Verification items for the finished model (mm, model axes). Face numbers are marked on the shaded views. A direction names the side the tool comes from. Give positions to 0.01 mm unless a question says otherwise; leave off trailing zeros. Order: outer loops, then holes, each group sorted by start corner. A loop starts at its lowest first (then second) coordinate and runs counter-clockwise, first axis right, second up. Notation, with made-up numbers: M -25,18 L 19,18 A24 ccw 19,45 Z; hole C 52.5,83 d1. An arc over 180 degrees is marked long. Answer as a JSON object with one key per item and string values.
```python
from build123d import *

# Parameters (mm, degrees)
SKETCH_R                       = 2.25
SKETCH_R_2                     = 1.75
PAD_DEPTH                      = 12
POCKET_DEPTH                   = 2
SKETCH002_R                    = 2.25
POCKET002_DEPTH                = 20.001
PART_MIRRORING_PLACEMENT_ANGLE = 180
SKETCH003_R                    = 3
POCKET003_DEPTH                = 8
SKETCH004_R                    = 3.75
POCKET004_DEPTH                = 10


with BuildPart() as pocket002:
    # Sketch → Pad (new body)
    with BuildSketch(Plane.XY):
        Polygon((0, -20), (40, -20), (40, 20), (-20, 20), (-20, 0), (0, 0), align=None)
        with Locations((18, 8)):
            Circle(SKETCH_R, mode=Mode.SUBTRACT)
        with Locations((13, -10)):
            Circle(SKETCH_R, mode=Mode.SUBTRACT)
        with Locations((35, 15)):
            Circle(SKETCH_R_2, mode=Mode.SUBTRACT)
        with Locations((28, -10)):
            Circle(SKETCH_R, mode=Mode.SUBTRACT)
    extrude(amount=PAD_DEPTH)

    # Sketch001 → Pocket (cut)
    with BuildSketch(Plane.XY.offset(12)):
        with BuildLine():
            Line((46, 10), (29, 10))
            ThreePointArc((29, 10), (25.778175, 17.778175), (18, 21))
            Line((18, 21), (0, 21))
            Line((0, 21), (0, -23))
            Line((0, -23), (46, -23))
            Line((46, -23), (46, -12))
            Line((28.629901, -14.455696), (46, -12))
            ThreePointArc((28.629901, -5.544304), (23.5, -10), (28.629901, -14.455696))
            Line((28.629901, -5.544304), (46, -8))
            Line((46, -8), (46, 10))
        make_face()
    extrude(amount=-POCKET_DEPTH, mode=Mode.SUBTRACT)

    # Sketch002 → Pocket002 (cut, through all)
    with BuildSketch(Plane.XZ):
        with Locations((-10, 6)):
            Circle(SKETCH002_R)
    extrude(amount=-POCKET002_DEPTH, mode=Mode.SUBTRACT)


with BuildPart() as pocket004:
    # Part__Mirroring: instance of Pocket002
    add(pocket002.part.mirror(Plane(origin=(10, -0.411961, 0), x_dir=(0, 1, 0), z_dir=(0, 0, 1))))


with BuildPart() as pocket004_1:
    # Part__Mirroring placement: moved
    add(pocket004.part.rotate(Axis((0, 0, 0), (1, 0, 0)), PART_MIRRORING_PLACEMENT_ANGLE))

    # Sketch003 → Pocket003 (cut)
    with BuildSketch(Plane(origin=(0, 0, 0), x_dir=(1, 0, 0), z_dir=(0, 0, -1))):
        with Locations((35, 15)):
            Circle(SKETCH003_R)
    extrude(amount=-POCKET003_DEPTH, mode=Mode.SUBTRACT)

    # Sketch004 → Pocket004 (cut)
    with BuildSketch(Plane(origin=(0, -20, 0), x_dir=(-1, 0, 0), z_dir=(0, -1, 0))):
        with Locations((10, -6)):
            Circle(SKETCH004_R)
    extrude(amount=-POCKET004_DEPTH, mode=Mode.SUBTRACT)


with BuildPart() as part_mirroring001:
    # Part__Mirroring001: instance of Pocket004
    add(pocket004_1.part.mirror(Plane(origin=(0, 0, 0), x_dir=(0, -1, 0), z_dir=(1, 0, 0))))


solid = part_mirroring001.part
```
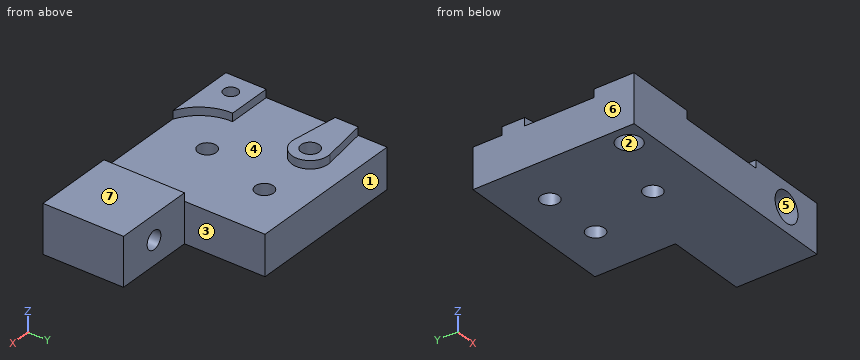
Q1. Section check B-B on y = 10. Record the cut outline in (x, z).
Resolved:
{"outline": "M -40,0 L -30.25,0 L -30.25,12 L -40,12 Z; M -25.75,0 L -15.25,0 L -15.25,10 L -23.5,10 L -23.5,12 L -25.75,12 Z; M -10.75,0 L 0,0 L 0,10 L -10.75,10 Z"}
Q2. Section check D-D on y = -8. Record the cut outline in (x, z).
Resolved:
{"outline": "M -40,0 L -20.25,0 L -20.25,10 L -40,10 Z; M -15.75,0 L 20,0 L 20,12 L 0,12 L 0,10 L -15.75,10 Z; hole C 10,6 d4.5"}
Q3. Gauge pin test, flat ends, axial feed: pin 1 Ø7 at (x, z) = (10, 6) entering from +Y; pin 2 Ø12 at (x, y) = (-25, -1) entering from +Z; pin 3 Ø3.5 at (x, z) = (10, 6) entering from +Y; pin 4 Ø3 at (y, z) = (13.5, 7.5) entering from +X. Record the tip position at first contact, or that the pin passes through.
Resolved:
{"pin 1": "stops at y = 0", "pin 2": "stops at z = 10", "pin 3": "passes through", "pin 4": "stops at x = 0"}
Q4. Tool access check on the marked faces 1, 2, 3 and 4. Record the directions out of +Z, -Z, +X, -X, +Y, -Y that give a thin tool (end or side, any length) a straight path to the whole face; none if there is none.
Resolved:
{"face 1": "+Z, -Z, +X, -X, +Y", "face 2": "-Z", "face 3": "+Z, -Z, +X, +Y", "face 4": "+Z"}
Q5. Section check C-C on x = -18. Record the cut outline in (y, z), then the cut area to 3 significant figures.
Resolved:
{"outline": "M -20,0 L -10.25,0 L -10.25,10 L -20,10 Z; M -5.75,0 L 20,0 L 20,10 L -5.75,10 Z", "area": "355 mm²"}
Q6. Section check A-A on z = 6. Record the cut outline in (x, y), then the cut area to 3 significant figures.
Resolved:
{"outline": "M -40,-20 L 6.25,-20 L 6.25,-10 L 7.75,-10 L 7.75,0 L 0,0 L 0,20 L -40,20 Z; M 12.25,-10 L 13.75,-10 L 13.75,-20 L 20,-20 L 20,0 L 12.25,0 Z; hole C -35,-15 d6; hole C -28,10 d4.5; hole C -18,-8 d4.5; hole C -13,10 d4.5", "area": "1,800 mm²"}
Q7. Release check for a two-part mould opening along Z. For the marked faces 5, 6 and 7 record: +Z half, -Z half, draft (parallel to the pull), parting line (faces both ways), or undercut.
Resolved:
{"face 5": "undercut", "face 6": "draft", "face 7": "+Z half"}
Q8. Material ranges on L1, parallel to X at y = 10, z = 4.5; L2, parallel to Y at x = -35, z = 5; L3, parallel to Y at x = -28, z = 3.5, recorded low to high.
Resolved:
{"L1": "x = -40 to -30.25, -25.75 to -15.25, -10.75 to 0", "L2": "y = -20 to -18, -12 to 20", "L3": "y = -20 to 7.75, 12.25 to 20"}
